from build123d import *

# Parameters (mm, degrees)
SKETCH1_W             = 0.68
SKETCH1_H             = 0.68
BOSS_EXTRUDE1_DEPTH   = 3.2
BOSS_EXTRUDE1_2_DEPTH = 3.2
BOSS_EXTRUDE1_3_DEPTH = 3.2
BOSS_EXTRUDE1_4_DEPTH = 3.2
BOSS_EXTRUDE1_5_DEPTH = 3.2
BOSS_EXTRUDE1_6_DEPTH = 3.2
BOSS_EXTRUDE1_7_DEPTH = 3.2
BOSS_EXTRUDE1_8_DEPTH = 3.2
BOSS_EXTRUDE1_9_DEPTH = 3.2
SKETCH2_W             = 32.8
SKETCH2_H             = 12.5
BOSS_EXTRUDE2_DEPTH   = 12.5
FILLET1_R             = 1
SKETCH3_W             = 10.5
SKETCH3_H             = 2.3
CUT_EXTRUDE1_DEPTH    = 37.369223253
SKETCH4_W             = 3.7
SKETCH4_H             = 0.68
BOSS_EXTRUDE3_DEPTH   = 4
CUT_EXTRUDE5_DEPTH    = 23.571716816
FILLET2_R             = 0.3
BOSS_EXTRUDE4_DEPTH   = 6.5
FILLET3_R             = 1
CUT_EXTRUDE6_DEPTH    = 6.5
FILLET4_R             = 3
SKETCH12_W            = 3
SKETCH12_H            = 9
CUT_EXTRUDE7_DEPTH    = 8
FILLET5_R             = 0.5


with BuildPart() as part:
    # Sketch1 → Boss-Extrude1 (new body)
    with BuildSketch(Plane(origin=(0, 0, 0), x_dir=(1, 0, 0), z_dir=(0, 1, 0))):
        with Locations((1.385, -1.42)):
            Rectangle(SKETCH1_W, SKETCH1_H)
    extrude(amount=-BOSS_EXTRUDE1_DEPTH)



with BuildPart() as body_2:
    # Sketch1 → Boss-Extrude1 2 (new body)
    with BuildSketch(Plane(origin=(0, 0, 0), x_dir=(1, 0, 0), z_dir=(0, 1, 0))):
        with Locations((-1.385, -1.42)):
            Rectangle(SKETCH1_W, SKETCH1_H)
    extrude(amount=-BOSS_EXTRUDE1_2_DEPTH)


with BuildPart() as body_3:
    # Sketch1 → Boss-Extrude1 3 (new body)
    with BuildSketch(Plane(origin=(0, 0, 0), x_dir=(1, 0, 0), z_dir=(0, 1, 0))):
        with Locations((-5.54, 1.42)):
            Rectangle(SKETCH1_W, SKETCH1_H)
    extrude(amount=-BOSS_EXTRUDE1_3_DEPTH)


with BuildPart() as body_4:
    # Sketch1 → Boss-Extrude1 4 (new body)
    with BuildSketch(Plane(origin=(0, 0, 0), x_dir=(1, 0, 0), z_dir=(0, 1, 0))):
        with Locations((-2.77, 1.42)):
            Rectangle(SKETCH1_W, SKETCH1_H)
    extrude(amount=-BOSS_EXTRUDE1_4_DEPTH)


with BuildPart() as body_5:
    # Sketch1 → Boss-Extrude1 5 (new body)
    with BuildSketch(Plane(origin=(0, 0, 0), x_dir=(1, 0, 0), z_dir=(0, 1, 0))):
        with Locations((-4.155, -1.42)):
            Rectangle(SKETCH1_W, SKETCH1_H)
    extrude(amount=-BOSS_EXTRUDE1_5_DEPTH)


with BuildPart() as body_6:
    # Sketch1 → Boss-Extrude1 6 (new body)
    with BuildSketch(Plane(origin=(0, 0, 0), x_dir=(1, 0, 0), z_dir=(0, 1, 0))):
        with Locations((0, 1.42)):
            Rectangle(SKETCH1_W, SKETCH1_H)
    extrude(amount=-BOSS_EXTRUDE1_6_DEPTH)


with BuildPart() as body_7:
    # Sketch1 → Boss-Extrude1 7 (new body)
    with BuildSketch(Plane(origin=(0, 0, 0), x_dir=(1, 0, 0), z_dir=(0, 1, 0))):
        with Locations((4.155, -1.42)):
            Rectangle(SKETCH1_W, SKETCH1_H)
    extrude(amount=-BOSS_EXTRUDE1_7_DEPTH)


with BuildPart() as body_8:
    # Sketch1 → Boss-Extrude1 8 (new body)
    with BuildSketch(Plane(origin=(0, 0, 0), x_dir=(1, 0, 0), z_dir=(0, 1, 0))):
        with Locations((5.54, 1.42)):
            Rectangle(SKETCH1_W, SKETCH1_H)
    extrude(amount=-BOSS_EXTRUDE1_8_DEPTH)


with BuildPart() as body_9:
    # Sketch1 → Boss-Extrude1 9 (new body)
    with BuildSketch(Plane(origin=(0, 0, 0), x_dir=(1, 0, 0), z_dir=(0, 1, 0))):
        with Locations((2.77, 1.42)):
            Rectangle(SKETCH1_W, SKETCH1_H)
    extrude(amount=-BOSS_EXTRUDE1_9_DEPTH)


with BuildPart() as part_1:
    add(part.part)

    add(body_2.part)  # Boss-Extrude2 merges body 2

    add(body_3.part)  # Boss-Extrude2 merges body 3

    add(body_4.part)  # Boss-Extrude2 merges body 4

    add(body_5.part)  # Boss-Extrude2 merges body 5

    add(body_6.part)  # Boss-Extrude2 merges body 6

    add(body_7.part)  # Boss-Extrude2 merges body 7

    add(body_8.part)  # Boss-Extrude2 merges body 8

    add(body_9.part)  # Boss-Extrude2 merges body 9
    # Sketch2 → Boss-Extrude2 (add)
    with BuildSketch(Plane(origin=(0, 0, 0), x_dir=(1, 0, 0), z_dir=(0, 1, 0))):
        with Locations((0, -3.27)):
            Rectangle(SKETCH2_W, SKETCH2_H)
    extrude(amount=BOSS_EXTRUDE2_DEPTH)

    # Fillet1
    fillet1_edges = [part_1.edges().sort_by_distance(p)[0] for p in [
        (-16.4, 0, 3.27),
        (16.4, 0, 3.27),
        (-16.4, 12.5, 3.27),
        (16.4, 12.5, 3.27),
    ]]
    fillet(fillet1_edges, radius=FILLET1_R)

    # Sketch3 → Cut-Extrude1 (cut, through all)
    with BuildSketch(Plane(origin=(16.4, 0, 0), x_dir=(0, 0, -1), z_dir=(1, 0, 0))):
        with Locations((-2.27, 11.35)):
            Rectangle(SKETCH3_W, SKETCH3_H)
    extrude(amount=-CUT_EXTRUDE1_DEPTH, mode=Mode.SUBTRACT)

    # Sketch4 → Boss-Extrude3 (add)
    with BuildSketch(Plane.XZ):
        with Locations((-12.495, 0)):
            Rectangle(SKETCH4_W, SKETCH4_H)
        with Locations((12.495, 0)):
            Rectangle(SKETCH4_W, SKETCH4_H)
    extrude(amount=BOSS_EXTRUDE3_DEPTH)

    # Sketch6 → Cut-Extrude5 (cut, through all)
    with BuildSketch(Plane.XY.offset(0.34)):
        Polygon((-14.345, -1.550750234), (-13.813289593, -0.780582126), (-13.813289593, 0), (-14.345, 0), (-14.827308736, 0), (-14.827308736, -4), (-13.896384817, -4), align=None)
        Polygon((-12.907050916, 0), (-12.082949084, 0), (-12.082949084, -3.533172452), (-11.651133602, -4), (-13.338866398, -4), (-12.907050916, -3.533172452), align=None)
        Polygon((-11.176710407, 0), (-10.645, 0), (-10.162691264, 0), (-10.162691264, -4), (-11.093615183, -4), (-10.645, -1.550750234), (-11.176710407, -0.780582126), align=None)
        Polygon((10.645, -1.550750234), (11.176710407, -0.780582126), (11.176710407, 0), (10.645, 0), (10.162691264, 0), (10.162691264, -4), (11.093615183, -4), align=None)
        Polygon((12.082949084, 0), (12.082949084, -3.533172452), (11.651133602, -4), (13.338866398, -4), (12.907050916, -3.533172452), (12.907050916, 0), align=None)
        Polygon((13.813289593, 0), (14.345, 0), (14.827308736, 0), (14.827308736, -4), (13.896384817, -4), (14.345, -1.550750234), (13.813289593, -0.780582126), align=None)
    extrude(amount=-CUT_EXTRUDE5_DEPTH, mode=Mode.SUBTRACT)

    # Fillet2
    fillet2_edges = [part_1.edges().sort_by_distance(p)[0] for p in [
        (13.896384817, -4, 0),
        (11.093615183, -4, 0),
        (11.651133602, -4, 0),
        (13.338866398, -4, 0),
        (-13.338866398, -4, 0),
        (-11.651133602, -4, 0),
        (-11.093615183, -4, 0),
        (-13.896384817, -4, 0),
    ]]
    fillet(fillet2_edges, radius=FILLET2_R)

    # Sketch7 → Boss-Extrude4 (add)
    with BuildSketch(Plane.XY.offset(9.52)):
        Polygon((-8.95, 10.85), (8.95, 10.85), (8.95, 9.82390435), (7.508720125, 1.65), (-7.508720125, 1.65), (-8.95, 9.82390435), align=None)
    extrude(amount=BOSS_EXTRUDE4_DEPTH)

    # Fillet3
    fillet3_edges = [part_1.edges().sort_by_distance(p)[0] for p in [
        (-8.95, 10.85, 12.77),
        (-7.508720125, 1.65, 12.77),
        (7.508720125, 1.65, 12.77),
        (8.95, 10.85, 12.77),
    ]]
    fillet(fillet3_edges, radius=FILLET3_R)

    # Sketch10 → Cut-Extrude6 (cut)
    with BuildSketch(Plane.XY.offset(16.02)):
        with BuildLine():
            Line((-8.625, 9.85), (-7.335651287, 2.540327837))
            ThreePointArc((-7.335651287, 2.540327837), (-7.106424964, 2.135386694), (-6.669620494, 1.975))
            Line((-6.669620494, 1.975), (6.669620494, 1.975))
            ThreePointArc((6.669620494, 1.975), (7.146917571, 2.172702923), (7.344620494, 2.65))
            Line((7.344620494, 2.65), (8.621293798, 9.779362644))
            ThreePointArc((8.621293798, 9.779362644), (8.451649886, 10.301633028), (7.95, 10.525))
            Line((7.95, 10.525), (-7.95, 10.525))
            ThreePointArc((-7.95, 10.525), (-8.427297077, 10.327297077), (-8.625, 9.85))
        make_face()
    extrude(amount=-CUT_EXTRUDE6_DEPTH, mode=Mode.SUBTRACT)

    # Fillet4
    fillet4_edges = [part_1.edges().sort_by_distance(p)[0] for p in [
        (-16.4, 10.2, 2.27),
        (16.4, 10.2, 2.27),
    ]]
    fillet(fillet4_edges, radius=FILLET4_R)

    # Sketch12 → Cut-Extrude7 (cut)
    with BuildSketch(Plane(origin=(0, 10.2, 0), x_dir=(1, 0, 0), z_dir=(0, 1, 0))):
        with Locations((-14.9, -1.52)):
            Rectangle(SKETCH12_W, SKETCH12_H)
        with Locations((14.9, -1.52)):
            Rectangle(SKETCH12_W, SKETCH12_H)
    extrude(amount=-CUT_EXTRUDE7_DEPTH, mode=Mode.SUBTRACT)

    # Fillet5
    fillet5_edges = [part_1.edges().sort_by_distance(p)[0] for p in [
        (0, 0, -2.98),
        (-16.107106781, 0.292893219, -2.98),
        (16.107106781, 0.292893219, -2.98),
        (0, 10.2, -2.98),
        (16.4, 1.6, -2.98),
        (-16.4, 1.6, -2.98),
        (-14.9, 2.2, -2.98),
        (-13.4, 6.2, -2.98),
        (14.9, 2.2, -2.98),
        (13.4, 6.2, -2.98),
    ]]
    fillet(fillet5_edges, radius=FILLET5_R)


solid = part_1.part
Geometry check sheet. Reference: the model listing, model coordinates, mm. A direction names the side the tool comes from. Round coordinates to 2 decimals unless told otherwise and drop trailing zeros. Write each loop counter-clockwise with the first axis right and the second up, starting at its lowest first coordinate (ties: lowest second). Pieces come first, ordered by that corner, then holes. Notation, with made-up numbers: (43, 43) - (88, 43) arc R9 cw to (88, 47) - close; hole circle Ø5 at (56, 39.25). An arc over 180 degrees is marked (long way). One line per item, written item: value.
1. Cross-section at D-D on z = 8. Record the boundary of the cut face in (x, y).
The answers:
outline: (-16.4, 1) arc R1 ccw to (-15.4, 0) - (15.4, 0) arc R1 ccw to (16.4, 1) - (16.4, 11.5) arc R1 ccw to (15.4, 12.5) - (-15.4, 12.5) arc R1 ccw to (-16.4, 11.5) - close
2. Cross-section at A-A on z = 10.75. Record the boundary of the cut face in (x, y) (3 decimals).
The answers:
outline: (-8.95, 9.824) - (-7.654, 2.476) arc R1 ccw to (-6.67, 1.65) - (6.67, 1.65) arc R1 ccw to (7.654, 2.476) - (8.95, 9.824) - (8.95, 9.85) arc R1 ccw to (7.95, 10.85) - (-7.95, 10.85) arc R1 ccw to (-8.95, 9.85) - close; hole (-8.625, 9.85) - (-7.336, 2.54) arc R0.675 ccw to (-6.67, 1.975) - (6.67, 1.975) arc R0.675 ccw to (7.345, 2.65) - (8.621, 9.779) arc R0.675 ccw to (7.95, 10.525) - (-7.95, 10.525) arc R0.675 ccw to start
3. Scan lines: L1, parallel to Y at x = -0.5, z = 15.25 (3 decimals); L2, parallel to Y at x = 6, z = 3.25; L3, parallel to Z at x = -6, y = 2.75. Record each from-to range of solid material in increasing order.
The answers:
L1: y = 1.65 to 1.975, 10.525 to 10.85
L2: y = 0 to 10.2
L3: z = -2.98 to 9.52
4. Cross-section at B-B on x = 0. Record the boundary of the cut face in (y, z) (3 decimals).
The answers:
outline: (-3.2, -1.76) - (0, -1.76) - (0, -2.48) arc R0.5 ccw to (0.5, -2.98) - (9.7, -2.98) arc R0.5 ccw to (10.2, -2.48) - (10.2, 7.52) - (12.5, 7.52) - (12.5, 9.52) - (10.85, 9.52) - (10.85, 16.02) - (10.525, 16.02) - (10.525, 9.52) - (1.975, 9.52) - (1.975, 16.02) - (1.65, 16.02) - (1.65, 9.52) - (0, 9.52) - (0, -1.08) - (-3.2, -1.08) - close
5. Set-up check for faces 4 (the face through (-7.305, 1.878, 12.816)), 5 (the face through (-13.5, -2, -0.34)), 6 (the face through (-13.5, -2, 0.34)), 7 (the face through (8.649, 10.565, 12.816)): record each of +Z, -Z, +X, -X, +Y, -Y from which the full face is reachable in a straight line by a thin tool's end or side.
The answers:
face 4: +Z, -X, -Y
face 5: -Z, +X, -X, -Y
face 6: +Z, +X, -X, -Y
face 7: +Z, +X, +Y
6. Cross-section at C-C on y = 9.25. Record the boundary of the cut face in (x, z), and give its area (3 significant figures).
The answers:
outline: (-16.4, 7.52) - (-15.59, 7.52) - (-15.59, 6.02) - (-13.4, 6.02) - (-13.4, -2.48) arc R0.5 ccw to (-12.9, -2.98) - (12.9, -2.98) arc R0.5 ccw to (13.4, -2.48) - (13.4, 6.02) - (15.59, 6.02) - (15.59, 7.52) - (16.4, 7.52) - (16.4, 9.52) - (8.85, 9.52) - (8.85, 16.02) - (8.53, 16.02) - (8.53, 9.52) - (-8.52, 9.52) - (-8.52, 16.02) - (-8.85, 16.02) - (-8.85, 9.52) - (-16.4, 9.52) - close
area: 358 mm^2
7. Mould release check, pull along Y, two halves, no side actions. Record for faces 1 (the face through (0, 10.525, 13)), 2 (the face through (8.31, 6.2, 12.72)), 3 (the face through (-15, 6, 6.02)): released by +Y, released by -Y, zero draft, split by the parting line, or undercut.
The answers:
face 1: undercut
face 2: released by -Y
face 3: zero draft
8. Depth check by flat-ended pin: pin 1 Ø2.5 at (x, y) = (-14.5, 8) entering from -Z; pin 2 Ø3 at (y, z) = (9.5, 0.5) entering from +X; pin 3 Ø1.2 at (x, y) = (-11.5, -1.5) entering from +Z. Enter the tip coordinate at first touch or a pass-through.
The answers:
pin 1: stops at z = -2.84
pin 2: stops at x = 13.4
pin 3: stops at z = 0.34
